For this review, take the finished solid that the model builds, in its own axes (mm). A direction names the side the tool comes from. Round coordinates to 2 decimals unless told otherwise and drop trailing zeros. Loops run counter-clockwise (first coordinate to the right, second up) from the corner with the lowest first, then second, coordinate; pieces in that order, holes last.
1. Consider section C-C on x = 30.5. State the section outline as (y, z) points, then the cut area to 3 significant figures.
2. Clearance check with a flat-ended pin moving along its axis: pin 1 Ø5 at (x, y) = (-30.16, 11.11) entering from +Z. State where the tip first meets the part, or that it passes through.
3. Tool access review of faces 5 (the flat face through (-6, -12, 4.762)), 6 (the cylindrical face through (27.013, -13.527, 12.522)): name each direction out of +Z, -Z, +X, -X, +Y, -Y from which nothing blocks a thin tool from reaching the whole face with its end or side.
4. To check wall thickness, follow line 1 along Y through (x, z) = (0, 2.6) (3 decimals); line 2 along Y through (x, z) = (28, 22); line 3 along Y through (x, z) = (29, 19.5). State the ranges of each line that lie inside material, in increasing order.
5. Consider section A-A on y = 0. State the section outline as (x, z) points (1 decimal).
6. Consider section D-D on z = 15.5. State the section outline as (x, y) points.
7. Draft analysis for pull direction Y (two halves, no side actions). For faces 1 (the flat face through (38.1, 0, 13)), 2 (the cylindrical face through (-33.312, 8.698, 12.522)), 3 (the flat face through (-1, -19.05, 13)), 4 (the cylindrical face through (-33.31, -13.53, 12.52)), state which applies: released by +Y, released by -Y, zero draft, split by the parting line, or undercut.
from build123d import *

# Parameters (mm, degrees)
F0_W         = 76.2
F0_H         = 38.1
F0_R         = 3.96875
F1_DEPTH     = 25.4
F2_R         = 0.381
F3_R         = 0.381
F4_T1_DEPTH  = 25.9715
F4_S5_W      = 0.381
F4_S5_H      = 0.381
F4_T6_DEPTH  = 0.381
F4_S11_W     = 0.381
F4_S11_H     = 0.381
F4_T12_DEPTH = 0.381
F5_R         = 12.7
F6_DEPTH     = 25.4
F7_R         = 15.875
F8_DEPTH     = 4.7625
F9_SIZE      = 0.381


# Not quite as in the source:
# - a fillet or chamfer that OpenCascade refuses, or shapes differently, is made with other operations: its cross-section is extruded or revolved along the edge and cut away or added


with BuildPart() as f1:
    # F0 (on Top) → F1 (new body)
    with BuildSketch(Plane.XY):
        Rectangle(F0_W, F0_H)
        with Locations((-30.1625, -11.1125)):
            Circle(F0_R, mode=Mode.SUBTRACT)
        with Locations((30.1625, -11.1125)):
            Circle(F0_R, mode=Mode.SUBTRACT)
        with Locations((-30.1625, 11.1125)):
            Circle(F0_R, mode=Mode.SUBTRACT)
        with Locations((30.1625, 11.1125)):
            Circle(F0_R, mode=Mode.SUBTRACT)
    extrude(amount=F1_DEPTH)

    # F2
    f2_edges = [f1.edges().sort_by_distance(p)[0] for p in [
        (0, -19.05, 0),
        (38.1, 0, 0),
        (-38.1, 0, 0),
    ]]
    fillet(f2_edges, radius=F2_R)

    # F3
    f3_edges = [f1.edges().sort_by_distance(p)[0] for p in [
        (0, 19.05, 0),
    ]]
    fillet(f3_edges, radius=F3_R)

    # F4: fillet of radius 0.381 on 3 edges, made by hand

    # F4_s2 → F4_t1 (cut)
    with BuildSketch(Plane.XY.offset(0.381)):
        with BuildLine():
            ThreePointArc((38.1, -18.669), (37.9884076836, -18.9384076836), (37.719, -19.05))
            Line((37.719, -19.05), (38.1, -19.05))
            Line((38.1, -19.05), (38.1, -18.669))
        make_face()
        with BuildLine():
            ThreePointArc((-37.719, -19.05), (-37.9884076836, -18.9384076836), (-38.1, -18.669))
            Line((-38.1, -18.669), (-38.1, -19.05))
            Line((-38.1, -19.05), (-37.719, -19.05))
        make_face()
    extrude(amount=F4_T1_DEPTH, mode=Mode.SUBTRACT)


with BuildPart() as f4_tool4:
    # F4_s5 → F4_t6 (new body)
    with BuildSketch(Plane.XZ.offset(18.669)):
        with Locations((-37.9095, 0.1905)):
            Rectangle(F4_S5_W, F4_S5_H)
    extrude(amount=F4_T6_DEPTH)

    # F4_s7 → F4_t8 (revolve, cut)
    with BuildSketch(Plane(origin=(-37.719, -18.669, 0.381), x_dir=(0.7071067812, 0, 0.7071067812), z_dir=(0.7071067812, 0, -0.7071067812))):
        with BuildLine():
            ThreePointArc((0, -0.381), (0.381, 0), (0, 0.381))
            Line((0, 0.381), (0, -0.381))
        make_face()
    revolve(axis=Axis((-37.719, -18.669, 0.381), (0, -1, 0)), mode=Mode.SUBTRACT)


with BuildPart() as f1_1:
    add(f1.part)

    # F4_t3: cut F4_tool4
    add(f4_tool4.part, mode=Mode.SUBTRACT)


with BuildPart() as f4_tool10:
    # F4_s11 → F4_t12 (new body)
    with BuildSketch(Plane.YZ.offset(37.719)):
        with Locations((-18.8595, 0.1905)):
            Rectangle(F4_S11_W, F4_S11_H)
    extrude(amount=F4_T12_DEPTH)

    # F4_s13 → F4_t14 (revolve, cut)
    with BuildSketch(Plane(origin=(37.719, -18.669, 0.381), x_dir=(0, 0.7071067812, 0.7071067812), z_dir=(0, 0.7071067812, -0.7071067812))):
        with BuildLine():
            ThreePointArc((0, -0.381), (0.381, 0), (0, 0.381))
            Line((0, 0.381), (0, -0.381))
        make_face()
    revolve(axis=Axis((37.719, -18.669, 0.381), (1, 0, 0)), mode=Mode.SUBTRACT)


with BuildPart() as f1_2:
    add(f1_1.part)

    # F4_t9: cut F4_tool10
    add(f4_tool10.part, mode=Mode.SUBTRACT)

    # F5 (on face) → F6 (cut)
    with BuildSketch(Plane.XY.offset(25.4)):
        Circle(F5_R)
    extrude(amount=-F6_DEPTH, mode=Mode.SUBTRACT)

    # F7 (on face) → F8 (cut)
    with BuildSketch(Plane(origin=(0, 0, 0), x_dir=(1, 0, 0), z_dir=(0, 0, -1))):
        Circle(F7_R)
    extrude(amount=-F8_DEPTH, mode=Mode.SUBTRACT)

    # F9
    f9_edges = [f1_2.edges().sort_by_distance(p)[0] for p in [
        (-12.7, 0, 4.7625),
    ]]
    chamfer(f9_edges, length=F9_SIZE)


solid = f1_2.part
Resolved:
1. outline: (-19.05, 0.38) arc R0.38 ccw to (-18.67, 0) - (-15.07, 0) - (-15.07, 25.4) - (-19.05, 25.4) - close; (-7.16, 0) - (7.16, 0) - (7.16, 25.4) - (-7.16, 25.4) - close; (15.07, 0) - (18.67, 0) arc R0.38 ccw to (19.05, 0.38) - (19.05, 25.4) - (15.07, 25.4) - close
1. area: 566 mm2
2. pin 1: passes through
3. face 5: -Z
3. face 6: +Z, -Z
4. line 1: y = -19.05 to -15.875, 15.875 to 19.05
4. line 2: y = -19.05 to -14.44, -7.78 to 7.78, 14.44 to 19.05
4. line 3: y = -19.05 to -14.91, -7.32 to 7.32, 14.91 to 19.05
5. outline: (-38.1, 0.4) arc R0.4 ccw to (-37.7, 0) - (-15.9, 0) - (-15.9, 4.8) - (-13.1, 4.8) - (-12.7, 5.1) - (-12.7, 25.4) - (-38.1, 25.4) - close; (12.7, 5.1) - (13.1, 4.8) - (15.9, 4.8) - (15.9, 0) - (37.7, 0) arc R0.4 ccw to (38.1, 0.4) - (38.1, 25.4) - (12.7, 25.4) - close
6. outline: (-38.1, -18.67) arc R0.38 ccw to (-37.72, -19.05) - (37.72, -19.05) arc R0.38 ccw to (38.1, -18.67) - (38.1, 18.67) arc R0.38 ccw to (37.72, 19.05) - (-37.72, 19.05) arc R0.38 ccw to (-38.1, 18.67) - close; hole circle Ø7.94 at (-30.16, -11.11); hole circle Ø7.94 at (-30.16, 11.11); hole circle Ø25.4 at (0, 0); hole circle Ø7.94 at (30.16, -11.11); hole circle Ø7.94 at (30.16, 11.11)
7. face 1: zero draft
7. face 2: undercut
7. face 3: released by -Y
7. face 4: undercut
